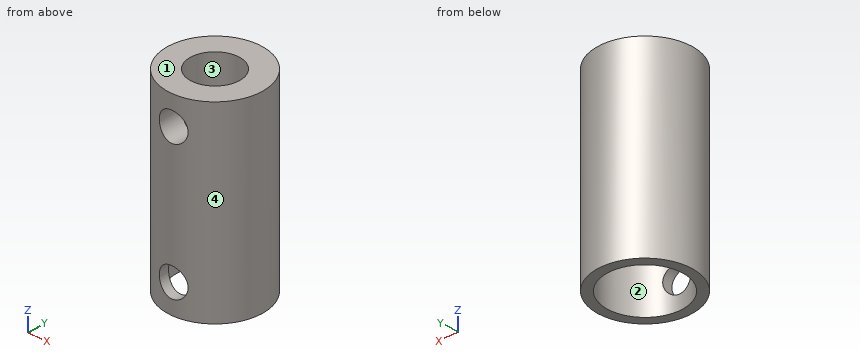
```python
from build123d import *

# Parameters (mm, degrees)
SKETCH1_R           = 10
BOSS_EXTRUDE1_DEPTH = 20
SKETCH5_R           = 8
CUT_EXTRUDE2_DEPTH  = 25
SKETCH6_R           = 5.2
CUT_EXTRUDE3_DEPTH  = 25
SKETCH7_R           = 3
CUT_EXTRUDE4_DEPTH  = 10


with BuildPart() as part:
    # Sketch1 → Boss-Extrude1 (new, symmetric)
    with BuildSketch(Plane.XY):
        Circle(SKETCH1_R)
    extrude(amount=BOSS_EXTRUDE1_DEPTH, both=True)

    # Sketch5 → Cut-Extrude2 (cut)
    with BuildSketch(Plane.XY):
        Circle(SKETCH5_R)
    extrude(amount=-CUT_EXTRUDE2_DEPTH, mode=Mode.SUBTRACT)

    # Sketch6 → Cut-Extrude3 (cut)
    with BuildSketch(Plane.XY):
        Circle(SKETCH6_R)
    extrude(amount=CUT_EXTRUDE3_DEPTH, mode=Mode.SUBTRACT)

    # Sketch7 → Cut-Extrude4 (cut)
    with BuildSketch(Plane(origin=(0, 0, 0), x_dir=(1, 0, 0), z_dir=(0, 1, 0))):
        with Locations(Location((0, 14, 0), (0, 0, 270))):
            Circle(SKETCH7_R)
        with Locations(Location((0, -14, 0), (0, 0, 270))):
            Circle(SKETCH7_R)
    extrude(amount=-CUT_EXTRUDE4_DEPTH, mode=Mode.SUBTRACT)


solid = part.part
```
Source: CAD feature listing. Evaluate the final solid. Frame: model axes, mm. Face numbers are marked on the shaded views. Round coordinates to 2 decimals unless told otherwise and drop trailing zeros. Loops run counter-clockwise (first coordinate to the right, second up) from the corner with the lowest first, then second, coordinate; pieces in that order, holes last. Notation, with made-up numbers: M -8,27 L 34,27 A31 cw 34,52 Z; hole C 65.5,-30.75 d1. An arc over 180 degrees is marked long. Use a Markdown table: item, result. Add a question column.
1. Pull-direction query (Y, two-part tool) for the marked faces 1, 2, 3 and 4; classes: +Y half, -Y half, draft (parallel to the pull), parting line (faces both ways), or undercut.
2. Cut plane B-B, the plane y = 0. Output: boundary loops of the cut face in (x, z), and give its area (3 significant figures).
3. Contact query for flat-ended pins moving along their axis: pin 1 (5 mm diameter, centred on x = 3.5, y = 1, fed in from -Z); pin 2 (5 mm diameter, centred on x = 0, z = -14, fed in from -Y); pin 3 (2 mm diameter, centred on x = -4, z = -12.5, fed in from +Y). Output: stop coordinate, or through.
4. Cut plane D-D, the plane z = -8. Output: boundary loops of the cut face in (x, y), and give its area (3 significant figures).
5. Cut plane C-C, the plane x = -4.25. Output: boundary loops of the cut face in (y, z), and give its area (3 significant figures).
6. Cut plane A-A, the plane x = 0. Output: boundary loops of the cut face in (y, z), and give its area (3 significant figures).
7. Ray query, line 1 along Y through (x, z) = (0, 6.25); line 2 along X through (y, z) = (-0.75, 14); line 3 along X through (y, z) = (3, 13). Return the intervals inside material, ascending. Write a range as [from, to].
Solution:
| question | item | result |
|---|---|---|
| 1 | face 1 | draft |
| 1 | face 2 | undercut |
| 1 | face 3 | undercut |
| 1 | face 4 | parting line |
| 2 | outline | M -10,-20 L -8,-20 L -8,0 L -5.2,0 L -5.2,20 L -10,20 Z; M 5.2,0 L 8,0 L 8,-20 L 10,-20 L 10,20 L 5.2,20 Z |
| 2 | area | 272 mm2 |
| 3 | pin 1 | stops at z = 0 |
| 3 | pin 2 | stops at y = 7.6 |
| 3 | pin 3 | stops at y = 9.54 |
| 4 | outline | C 0,0 d20; hole C 0,0 d16 |
| 4 | area | 113 mm2 |
| 5 | outline | M -9.05,-20 L -6.78,-20 L -6.78,0 L -3,0 L -3,20 L -9.05,20 Z; M 3,0 L 6.78,0 L 6.78,-20 L 9.05,-20 L 9.05,20 L 3,20 Z |
| 5 | area | 333 mm2 |
| 6 | outline | M -10,-20 L -8,-20 L -8,-17 L -10,-17 Z; M -10,-11 L -8,-11 L -8,0 L -5.2,0 L -5.2,11 L -10,11 Z; M -10,17 L -5.2,17 L -5.2,20 L -10,20 Z; M 5.2,0 L 8,0 L 8,-20 L 10,-20 L 10,20 L 5.2,20 Z |
| 6 | area | 231 mm2 |
| 7 | line 1 | y = [-10, -5.2], [5.2, 10] |
| 7 | line 2 | x = [-9.97, -5.15], [5.15, 9.97] |
| 7 | line 3 | x = [-9.54, -4.25], [4.25, 9.54] |
